For this review, take the finished solid that the model builds, in its own axes (mm). A direction names the side the tool comes from. Coordinates: 2 decimals unless noted, no trailing zeros. Loops run counter-clockwise (first coordinate to the right, second up) from the corner with the lowest first, then second, coordinate; pieces in that order, holes last. Notation, with made-up numbers: (-23, 20.25) - (25, 20.25) arc R33 cw to (25, 59.25) - close; hole circle Ø10 at (57, -32). An arc over 180 degrees is marked (long way). One line per item, written item: value. Start each with the question number.
1. The part is to be moulded in two halves that separate along Y. For faces 1 (the face through (-1.44, 24.5, -0.03)), 2 (the face through (0.66, 23.01, 2.1)), 3 (the face through (-0.02, 14.64, 1.75)), 4 (the face through (1.897, 5.851, 6.024)), say which applies: released by +Y, released by -Y, zero draft, split by the parting line, or undercut.
2. For faces 5 (the face through (1.54, 5.96, 4.88)), 6 (the face through (0, 0, 0)), list the 3-axis set-ups (+Z, -Z, +X, -X, +Y, -Y) from which the entire face can be reached by the end or side of a thin tool; tool diameter is ignored.
3. Take a section at D-D, the plane y = 18.25. State the section outline as (x, z) points.
4. Insertion check: pin 1 (0.7 mm diameter, centred on y = 10.5, z = 0.5, fed in from +X); pin 2 (3 mm diameter, centred on x = 3, y = 21, fed in from +Z) (3 decimals); pin 3 (1 mm diameter, centred on x = -2.5, y = 13.5, fed in from -Z). Each pin has a flat end and moves straight along its axis. Give the tip position at first contact, or say it passes through.
5. Take a section at B-B, the plane x = 0. State the section outline as (y, z) points.
6. To check wall thickness, follow line 1 (Z direction, x = -0.5, y = 1.5); line 2 (Z direction, x = 2, y = 9); line 3 (X direction, y = 9.25, z = 1.5) (3 decimals). State the ranges of each line that lie inside material, in increasing order. Write a range as from..to.
7. Take a section at C-C, the plane y = 3.5. State the section outline as (x, z) points.
8. Take a section at A-A, the plane z = 0. State the section outline as (x, y) points, and give its area (3 significant figures).
Autodesk Inventor part; units mm, degrees
ref_plane "YZ Plane" through (0, 0, 0) normal (1, 0, 0) x (0, 1, 0)
ref_plane "XZ Plane" through (0, 0, 0) normal (0, 1, 0) x (-1, 0, 0)
ref_plane "XY Plane" through (0, 0, 0) normal (0, 0, 1) x (1, 0, 0)
sketch "Эскиз1" plane through (0, 0, 0) normal (1, 0, 0) x (0, 1, 0)
  line L0 (0, 0) -> (35, 0)
  line L1 (0, 0) -> (0, 6.15)
  line L2 (0, 6.15) -> (10.5958, 6.45)
  line L3 (10.5958, 6.45) -> (10.5958, 5.25)
  line L4 (10.5958, 5.25) -> (1.2, 4.984)
  line L5 (1.2, 4.984) -> (1.2, 2.7)
  line L6 (24.5, 2.7) -> (24.5, 0)
  line L7 (22.5, 2.7) -> (22.5, 2.2)
  line L8 (22.5, 2.2) -> (23.5, 2.2)
  line L9 (23.5, 2.2) -> (23.5, 2.7)
  line L10 (24.5, 2.7) -> (23.5, 2.7)
  line L11 (22.5, 2.7) -> (1.2, 2.7)
  point P0 (0, 3.075)
  dimension "d0" = 35
  dimension "d1" = 6.15
  dimension "d2" = 10.6
  dimension "d4" = 24.5
  dimension "d5" = 2.7
  dimension "d6" = 6.45
  dimension "d7" = 1.2
  dimension "d8" = 1.2
  dimension "d11" = 1
  dimension "d12" = 1
  dimension "d21" = 0.5
  dimension "d22" = 0
revolve "Вращение1" add sketch "Эскиз1" angle 360 about axis through (0, 0, 0) along (0, 1, 0)
fillet "Сопряжение1" radius 1 1 edges at (0, 0, -6.15)
sketch "Эскиз2" plane through (0, 24.5, 0) normal (0, 1, 0) x (1, 0, 0)
  circle A0 centre (0, 0) radius 1.75
  line L0 (-1.25, 1.2247) -> (-1.25, -1.2247)
  line L1 (1.25, 1.2247) -> (1.25, -1.2247)
  dimension "d13" = 3.5
  dimension "d19" = 1.25
  dimension "d20" = 1.25
extrude "Выдавливание1" cut sketch "Эскиз2" against normal blind 20 contours L1 A0 L0
chamfer "Фаска1" distance 0.5 angle 45 1 edges at (0, 24.5, -2.7)
properties part number "Кнопка для кухонной плиты"
Solutions:
1. face 1: released by +Y
1. face 2: undercut
1. face 3: zero draft
1. face 4: released by -Y
2. face 5: +Y
2. face 6: +Z, -Z, +X, -X, -Y
3. outline: circle Ø5.4 at (0, 0); hole (-1.25, -1.22) arc R1.75 ccw to (1.25, -1.22) - (1.25, 1.22) arc R1.75 ccw to (-1.25, 1.22) - close
4. pin 1: x = 6.45
4. pin 2: z = 2.245
4. pin 3: z = -1.81
5. outline: (0, -5.18) arc R1 ccw to (0.97, -6.18) - (10.6, -6.45) - (10.6, -5.25) - (1.2, -4.98) - (1.2, -2.7) - (22.5, -2.7) - (22.5, -2.2) - (23.5, -2.2) - (23.5, -2.7) - (24, -2.7) - (24.5, -2.2) - (24.5, -1.75) - (4.5, -1.75) - (4.5, 1.75) - (24.5, 1.75) - (24.5, 2.2) - (24, 2.7) - (23.5, 2.7) - (23.5, 2.2) - (22.5, 2.2) - (22.5, 2.7) - (1.2, 2.7) - (1.2, 4.98) - (10.6, 5.25) - (10.6, 6.45) - (0.97, 6.18) arc R1 ccw to (0, 5.18) - close
6. line 1: -6.17..-4.97, -2.65..2.65, 4.97..6.17
6. line 2: -6.08..-4.81, -1.81..1.81, 4.81..6.08
6. line 3: -6.234..-4.991, -2.245..-0.901, 0.901..2.245, 4.991..6.234
7. outline: circle Ø12.5 at (0, 0); circle Ø5.4 at (0, 0); hole circle Ø10.1 at (0, 0)
8. outline: (-6.45, 10.6) - (-6.18, 0.97) arc R1 ccw to (-5.18, 0) - (5.18, 0) arc R1 ccw to (6.18, 0.97) - (6.45, 10.6) - (5.25, 10.6) - (4.98, 1.2) - (2.7, 1.2) - (2.7, 22.5) - (2.2, 22.5) - (2.2, 23.5) - (2.7, 23.5) - (2.7, 24) - (2.2, 24.5) - (1.25, 24.5) - (1.25, 4.5) - (-1.25, 4.5) - (-1.25, 24.5) - (-2.2, 24.5) - (-2.7, 24) - (-2.7, 23.5) - (-2.2, 23.5) - (-2.2, 22.5) - (-2.7, 22.5) - (-2.7, 1.2) - (-4.98, 1.2) - (-5.25, 10.6) - close
8. area: 112 mm2
